```python
from build123d import *

# Parameters (mm, degrees)
SKETCH1_R           = 7.5
BOSS_EXTRUDE1_DEPTH = 1.57
SKETCH2_R           = 2.815
BOSS_EXTRUDE2_DEPTH = 19
SKETCH4_R           = 7
BOSS_EXTRUDE3_DEPTH = 0.8


with BuildPart() as part:
    # Sketch1 → Boss-Extrude1 (new body)
    with BuildSketch(Plane(origin=(0, 0, 0), x_dir=(1, 0, 0), z_dir=(0, 1, 0))):
        with Locations(Location((0, 0, 0), (0, 0, 270))):
            Circle(SKETCH1_R)
    extrude(amount=BOSS_EXTRUDE1_DEPTH)

    # Sketch2 → Boss-Extrude2 (add)
    with BuildSketch(Plane(origin=(0, 1.57, 0), x_dir=(1, 0, 0), z_dir=(0, 1, 0))):
        with Locations(Location((0, 0, 0), (0, 0, 270))):
            Circle(SKETCH2_R)
    extrude(amount=BOSS_EXTRUDE2_DEPTH)

    # Sketch3 → Revolve1 (revolve)
    with BuildSketch(Plane(origin=(0, 20.57, 0), x_dir=(1, 0, 0), z_dir=(0, 1, 0))):
        with BuildLine():
            Line((0, 6.35), (0, -6.35))
            ThreePointArc((0, -6.35), (6.35, 0), (0, 6.35))
        make_face()
    revolve(axis=Axis((0, 20.57, -8.311953328), (0, 0, 1)))

    # Sketch4 → Boss-Extrude3 (add)
    with BuildSketch(Plane.XZ):
        with Locations(Location((0, 0, 0), (0, 0, 270))):
            Circle(SKETCH4_R)
    extrude(amount=BOSS_EXTRUDE3_DEPTH)


solid = part.part
```
Work out the finished part from the listing and answer in its coordinate system (mm). Give positions to 0.01 mm unless a question says otherwise; leave off trailing zeros. Order: outer loops, then holes, each group sorted by start corner. A loop starts at its lowest first (then second) coordinate and runs counter-clockwise, first axis right, second up.
1. Section C-C, the plane x = 0 is taken. Determine the outline of the cut face in (y, z) (3 decimals).
Result sheet:
outline: (-0.8, -7) - (0, -7) - (0, -7.5) - (1.57, -7.5) - (1.57, -2.815) - (14.878, -2.815) arc R6.35 ccw (long way) to (14.878, 2.815) - (1.57, 2.815) - (1.57, 7.5) - (0, 7.5) - (0, 7) - (-0.8, 7) - close
2. Section D-D, the plane z = -1.25 is taken. Determine the outline of the cut face in (x, y), and give its area (3 significant figures).
Result sheet:
outline: (-7.4, 0) - (-6.89, 0) - (-6.89, -0.8) - (6.89, -0.8) - (6.89, 0) - (7.4, 0) - (7.4, 1.57) - (2.52, 1.57) - (2.52, 14.88) arc R6.23 ccw (long way) to (-2.52, 14.88) - (-2.52, 1.57) - (-7.4, 1.57) - close
area: 221 mm2
3. The mould has two halves that part along Y. Classify faces 1 (the flat face through (0, 1.57, 3)), 2 (the cylindrical face through (-6.834, -0.394, 1.517)), 3 (the cylindrical face through (2.79, 8.13, -0.37)), 4 (the flat face through (-7, 0, -2)): released by +Y, released by -Y, zero draft, split by the parting line, or undercut.
Result sheet:
face 1: undercut
face 2: zero draft
face 3: undercut
face 4: released by -Y
4. Straight lines are drawn through the part: L1, parallel to Y at x = 2, z = 6.25; L2, parallel to Y at x = -4, z = 4.5; L3, parallel to Y at x = 2.75, z = -1.75. For each, find the intervals that lie inside material, in ascending order.
Result sheet:
L1: y = -0.8 to 1.57
L2: y = -0.8 to 1.57, 18.55 to 22.59
L3: y = -0.8 to 1.57, 15.12 to 26.02
5. Each of these flat-tipped pins is pushed along its axis until it touches: P1, Ø8, axis at x = 0.5, y = 15.5, coming from the -Z side; P2, Ø2, axis at x = 1, z = -6, coming from the +Y side; P3, Ø2, axis at x = -3.5, z = 4, coming from the +Y side. Where does it stop, or does it pass through?
Result sheet:
P1: stops at z = -6.25
P2: stops at y = 24.38
P3: stops at y = 25.23
6. Section B-B, the plane z = 4.25 is taken. Determine the outline of the cut face in (x, y), and give its area (3 significant figures).
Result sheet:
outline: (-6.18, 0) - (-5.56, 0) - (-5.56, -0.8) - (5.56, -0.8) - (5.56, 0) - (6.18, 0) - (6.18, 1.57) - (-6.18, 1.57) - close; circle Ø9.44 at (0, 20.57)
area: 98.2 mm2
7. Section A-A, the plane x = -4.25 is taken. Determine the outline of the cut face in (y, z), and give its area (3 significant figures).
Result sheet:
outline: (-0.8, -5.56) - (0, -5.56) - (0, -6.18) - (1.57, -6.18) - (1.57, 6.18) - (0, 6.18) - (0, 5.56) - (-0.8, 5.56) - close; circle Ø9.44 at (20.57, 0)
area: 98.2 mm2
